Geometry check sheet. Reference: the model listing, model coordinates, mm. A direction names the side the tool comes from. Coordinates: 2 decimals unless noted, no trailing zeros. Order: outer loops, then holes, each group sorted by start corner. A loop starts at its lowest first (then second) coordinate and runs counter-clockwise, first axis right, second up. Notation, with made-up numbers: (-3, -20.75) - (8, -20.75) arc R25 cw to (8, 10.25) - close; hole circle Ø11 at (-38, -33). An arc over 180 degrees is marked (long way). Return JSON: item names as keys, results as strings. Group by question number.
Item 1: Gauge pin test, flat end, axial feed: pin 1 (5 mm diameter, centred on x = 5.5, z = 6, fed in from +Y). Record the tip position at first contact, or that the pin passes through.
Item 2: Section check C-C on x = 6.75. Enter the section's corners in (y, z), then the cut area to 3 significant figures.
Item 3: Section check D-D on y = 1.45. Enter the section's corners in (x, z), then the cut area to 3 significant figures.
Item 4: Scan lines: probe 1 along Y at (x, z) = (7.75, 1.75); probe 2 along Y at (x, z) = (0, 3); probe 3 along X at (y, z) = (0.4, 5.25). Record each from-to range of solid material in increasing order.
Item 5: Section check B-B on x = 8. Enter the section's corners in (y, z), then the cut area to 3 significant figures.
Item 6: Section check A-A on z = 5. Enter the section's corners in (x, y).
Item 7: Tool access check on faces 1 (the flat face through (3, -2, 0)), 2 (the flat face through (3.8, 0.1, 5.1)). Record the directions out of +Z, -Z, +X, -X, +Y, -Y that give a thin tool (end or side, any length) a straight path to the whole face; none if there is none.
Item 8: Draft check along X on faces 3 (the cylindrical face through (6.22, 0.61, 3.29)), 4 (the flat face through (4, 1.1, 4)), 5 (the flat face through (9, 0.6, 4.9)), 6 (the cylindrical face through (-1.61, 1.01, 4.93)). Enter one of: pulls with the +X half, pulls with the -X half, needs draft (parallel to the pull), parting line crosses it, or undercut.
from build123d import *

# Parameters (mm, degrees)
F0_R     = 1.9
F1_DEPTH = 10
F2_W     = 8.151472
F2_H     = 1.8
F3_DEPTH = 25
F4_R     = 1.75
F5_DEPTH = 25


with BuildPart() as f1:
    # F0 (on Top) → F1 (new body)
    with BuildSketch(Plane.XY):
        with BuildLine():
            ThreePointArc((0, -2.9), (2.05061, -2.05061), (2.9, 0))
            ThreePointArc((2.9, 0), (2.845305, 0.560573), (2.683282, 1.1))
            ThreePointArc((2.683282, 1.1), (-2.408319, 1.615549), (0, -2.9))
        make_face()
        Circle(F0_R, mode=Mode.SUBTRACT)
        with BuildLine():
            ThreePointArc((2.683282, 1.1), (2.845305, 0.560573), (2.9, 0))
            ThreePointArc((2.9, 0), (2.05061, -2.05061), (0, -2.9))
            Line((0, -2.9), (9, -2.9))
            Line((9, -2.9), (9, 1.1))
            Line((9, 1.1), (2.683282, 1.1))
        make_face()
    extrude(amount=F1_DEPTH)

    # F2 (on face) → F3 (cut)
    with BuildSketch(Plane.XY.offset(10)):
        with Locations((4.924264, -0.8)):
            Rectangle(F2_W, F2_H)
    extrude(amount=-F3_DEPTH, mode=Mode.SUBTRACT)

    # F4 (on face) → F5 (cut)
    with BuildSketch(Plane(origin=(0, 1.1, 0), x_dir=(-1, 0, 0), z_dir=(0, 1, 0))):
        with Locations((-5.841641, 5)):
            Circle(F4_R)
    extrude(amount=-F5_DEPTH, mode=Mode.SUBTRACT)


solid = f1.part
Computed:
{
 "1": {"pin 1": "stops at y = 1.1"},
 "2": {"outline": "(-2.9, 0) - (-1.7, 0) - (-1.7, 3.5) - (-2.9, 3.5) - close; (-2.9, 6.5) - (-1.7, 6.5) - (-1.7, 10) - (-2.9, 10) - close; (0.1, 0) - (1.1, 0) - (1.1, 3.5) - (0.1, 3.5) - close; (0.1, 6.5) - (1.1, 6.5) - (1.1, 10) - (0.1, 10) - close", "area": "15.4 mm²"},
 "3": {"outline": "(-2.51, 0) - (-1.23, 0) - (-1.23, 10) - (-2.51, 10) - close; (1.23, 0) - (2.51, 0) - (2.51, 10) - (1.23, 10) - close", "area": "25.7 mm²"},
 "4": {"probe 1": "y = -2.9 to -1.7, 0.1 to 1.1", "probe 2": "y = -2.9 to -1.9, 1.9 to 2.9", "probe 3": "x = -2.87 to -1.86, 1.86 to 4.11, 7.57 to 9"},
 "5": {"outline": "(-2.9, 0) - (-1.7, 0) - (-1.7, 10) - (-2.9, 10) - close; (0.1, 0) - (1.1, 0) - (1.1, 10) - (0.1, 10) - close", "area": "22.0 mm²"},
 "6": {"outline": "(0, -2.9) - (4.09, -2.9) - (4.09, -1.7) - (0.85, -1.7) arc R1.9 cw (long way) to (1.9, 0.1) - (4.09, 0.1) - (4.09, 1.1) - (2.68, 1.1) arc R2.9 ccw (long way) to start; (7.59, -2.9) - (9, -2.9) - (9, -1.7) - (7.59, -1.7) - close; (7.59, 0.1) - (9, 0.1) - (9, 1.1) - (7.59, 1.1) - close"},
 "7": {"face 1": "-Z, +X, -X, +Y, -Y", "face 2": "+Z, -Z, +X"},
 "8": {"face 3": "undercut", "face 4": "needs draft", "face 5": "pulls with the +X half", "face 6": "undercut"}
}
